Geometry check sheet. Reference: the model listing, model coordinates, mm. Round coordinates to 2 decimals unless told otherwise and drop trailing zeros. Write each loop counter-clockwise with the first axis right and the second up, starting at its lowest first coordinate (ties: lowest second). Pieces come first, ordered by that corner, then holes. Notation, with made-up numbers: M 63,13 L 113,13 A13 ccw 113,38 Z; hole C 9,21.25 d5. An arc over 180 degrees is marked long. One line per item, written item: value. Start each with the question number.
1. Section check A-A (y = 34.5). Record the boundary of the cut face in (x, z), and give its area (3 significant figures).
2. Scan lines: probe 1 along Z at (x, y) = (52, 18); probe 2 along Z at (x, y) = (69.5, 87.5). Record each from-to range of solid material in increasing order. Write a range as [from, to].
3. Section check B-B (x = 85). Record the boundary of the cut face in (y, z).
4. Depth check by flat-ended pin: P1, Ø10, axis at x = 45.5, z = 1898, coming from the -Y side; P2, Ø1.5, axis at x = 19, y = 49, coming from the +Z side; P3, Ø3, axis at x = 81, y = 31, coming from the +Z side; P4, Ø10, axis at x = 70.5, y = 51.5, coming from the +Z side. Enter the tip coordinate at first touch or a pass-through.
from build123d import *

# Parameters (mm, degrees)
F0_W     = 101.6
F0_H     = 101.6
F1_DEPTH = 3048
F3_DEPTH = 101.601
F5_DEPTH = 101.601
F7_DEPTH = 101.601


with BuildPart() as f1:
    # F0 (on Top) → F1 (new body)
    with BuildSketch(Plane.XY):
        with Locations((50.8, 50.8)):
            Rectangle(F0_W, F0_H)
    extrude(amount=F1_DEPTH)

    # F2 (on Front) → F3 (cut, through all)
    with BuildSketch(Plane.XZ):
        Polygon((101.6, 42.0840979371), (0, 0), (101.6, 0), align=None)
    extrude(amount=-F3_DEPTH, mode=Mode.SUBTRACT)

    # F4 (on face) → F5 (cut, through all)
    with BuildSketch(Plane.XZ):
        Polygon((0, 3048), (0, 2639.314), (101.6, 2681.3980979371), (101.6, 3048), align=None)
    extrude(amount=-F5_DEPTH, mode=Mode.SUBTRACT)

    # F6 (on face) → F7 (cut, through all)
    with BuildSketch(Plane.XZ):
        Polygon((101.6, 2681.3980979371), (43.2856477874, 2657.2435023697), (101.6, 2516.460202377), align=None)
    extrude(amount=-F7_DEPTH, mode=Mode.SUBTRACT)


solid = f1.part
Result sheet:
1. outline: M 0,0 L 101.6,42.08 L 101.6,2516.46 L 43.29,2657.24 L 0,2639.31 Z
1. area: 263,000 mm2
2. probe 1: z = [21.54, 2636.21]
2. probe 2: z = [28.79, 2593.96]
3. outline: M 0,35.21 L 101.6,35.21 L 101.6,2556.54 L 0,2556.54 Z
4. P1: stops at y = 0
4. P2: stops at z = 2647.49
4. P3: stops at z = 2569.81
4. P4: stops at z = 2603.61
